Work out the finished part from the listing and answer in its coordinate system (mm). A direction names the side the tool comes from. Give positions to 0.01 mm unless a question says otherwise; leave off trailing zeros. Write each loop counter-clockwise with the first axis right and the second up, starting at its lowest first coordinate (ties: lowest second). Pieces come first, ordered by that corner, then holes. Notation, with made-up numbers: (22, 76.25) - (33, 76.25) arc R8 ccw to (33, 90.25) - close; hole circle Ø5 at (73.25, 3.25). An arc over 180 degrees is marked (long way). Write item = value, one per line.
from build123d import *

# Parameters (mm, degrees)
ESBO_O1_W             = 50
ESBO_O1_H             = 50
BASE_DEPTH            = 3
ENTRADASESB_R         = 2
ENTRADASESB_W         = 31.12
ENTRADASESB_H         = 12.13
CORTE_EXTRUS_O1_DEPTH = 3


with BuildPart() as part:
    # Esboço1 → Base (new body)
    with BuildSketch(Plane(origin=(0, 0, 0), x_dir=(1, 0, 0), z_dir=(0, 1, 0))):
        with Locations((25, 25)):
            Rectangle(ESBO_O1_W, ESBO_O1_H)
    extrude(amount=BASE_DEPTH)

    # EntradasEsb → Corte-extrusão1 (cut)
    with BuildSketch(Plane(origin=(0, 3, 0), x_dir=(1, 0, 0), z_dir=(0, 1, 0))):
        with Locations(Location((25, 41.065, 0), (0, 0, 270))):
            Circle(ENTRADASESB_R)
        with Locations(Location((25, 8.935, 0), (0, 0, 270))):
            Circle(ENTRADASESB_R)
        with Locations(Location((44.56, 25, 0), (0, 0, 270))):
            Circle(ENTRADASESB_R)
        with Locations(Location((5.44, 25, 0), (0, 0, 270))):
            Circle(ENTRADASESB_R)
        with Locations((25, 25)):
            Rectangle(ENTRADASESB_W, ENTRADASESB_H)
    extrude(amount=-CORTE_EXTRUS_O1_DEPTH, mode=Mode.SUBTRACT)


solid = part.part
1. Straight lines are drawn through the part: line 1 (X direction, y = 1.2, z = -25); line 2 (Z direction, x = 31.5, y = 0.55) (3 decimals); line 3 (X direction, y = 1.2, z = -28). For each, find the intervals that lie inside material, in ascending order.
Solution:
line_1 = 0 to 3.44, 7.44 to 9.44, 40.56 to 42.56, 46.56 to 50
line_2 = -50 to -31.065, -18.935 to 0
line_3 = 0 to 9.44, 40.56 to 50
2. Find section C-C, the plane x = 25. Give the vertices of the cut face in (y, z) (3 decimals), then the cut area to 3 significant figures.
Solution:
outline = (0, -50) - (3, -50) - (3, -43.065) - (0, -43.065) - close; (0, -39.065) - (3, -39.065) - (3, -31.065) - (0, -31.065) - close; (0, -18.935) - (3, -18.935) - (3, -10.935) - (0, -10.935) - close; (0, -6.935) - (3, -6.935) - (3, 0) - (0, 0) - close
area = 89.6 mm^2
3. A tool of negligible diameter and unlimited length cuts with its end or side. For faces 5 (the flat face through (25, 1, -50)), 6 (the flat face through (25, 2, -18.935)), from which of +Z, -Z, +X, -X, +Y, -Y can it reach the whole face along a straight path? Write none if from no direction.
Solution:
face_5 = -Z, +X, -X, +Y, -Y
face_6 = +Y, -Y
4. Find section D-D, the plane x = 5.44. Give the vertices of the cut face in (y, z), then the cut area to 3 significant figures.
Solution:
outline = (0, -50) - (3, -50) - (3, -27) - (0, -27) - close; (0, -23) - (3, -23) - (3, 0) - (0, 0) - close
area = 138 mm^2
5. Find section B-B, the plane z = -25. Give the vertices of the cut face in (x, y).
Solution:
outline = (0, 0) - (3.44, 0) - (3.44, 3) - (0, 3) - close; (7.44, 0) - (9.44, 0) - (9.44, 3) - (7.44, 3) - close; (40.56, 0) - (42.56, 0) - (42.56, 3) - (40.56, 3) - close; (46.56, 0) - (50, 0) - (50, 3) - (46.56, 3) - close
6. Find section A-A, the plane y = 1.45. Give the vertices of the cut face in (x, z) (3 decimals), then the cut area to 3 significant figures.
Solution:
outline = (0, -50) - (50, -50) - (50, 0) - (0, 0) - close; hole circle Ø4 at (5.44, -25); hole (9.44, -31.065) - (40.56, -31.065) - (40.56, -18.935) - (9.44, -18.935) - close; hole circle Ø4 at (25, -41.065); hole circle Ø4 at (25, -8.935); hole circle Ø4 at (44.56, -25)
area = 2,070 mm^2
7. For a pull along Z with two mould halves and no side action, classify faces 1 (the flat face through (9.44, 2, -25)), 2 (the flat face through (25, 3, -36)), 3 (the flat face through (25, 1, 0)), 4 (the cylindrical face through (5.5, 1.5, -27)) as pulls with the +Z half, pulls with the -Z half, needs draft (parallel to the pull), parting line crosses it, or undercut.
Solution:
face_1 = undercut
face_2 = needs draft
face_3 = pulls with the +Z half
face_4 = undercut
